Can you work these out from the model? Positions are in its coordinate system, mm. A direction names the side the tool comes from. Coordinates: 2 decimals unless noted, no trailing zeros. Loops run counter-clockwise (first coordinate to the right, second up) from the corner with the lowest first, then second, coordinate; pieces in that order, holes last. Notation, with made-up numbers: M -5.5,83 L 27.5,83 A22 ccw 27.5,112 Z; hole C 49,80.25 d11. An arc over 180 degrees is marked long. Answer as a JSON object with one key per item and string values. Group by question number.
Item 1: Suppose I cut it at A-A (y = 20). Write out the boundary of the cut face in (x, z).
Item 2: Which directions (+Z, -Z, +X, -X, +Y, -Y) give clear straight access to the entire face, cutting with the end or side of a thin tool? Please do faces 4 (the cylindrical face through (127.502, 170.354, -59.79)), 5 (the flat face through (220.5, 142, -60)), 6 (the cylindrical face through (414.343, 143.385, 10.77)).
Item 3: I'm going to push flat-ended pins straight in: pin 1 Ø11 at (x, y) = (260.5, 174.5) entering from +Z; pin 2 Ø6 at (x, y) = (451.5, 139) entering from +Z; pin 3 Ø2.5 at (x, y) = (231, 140.5) entering from -Z. Where does each tip first touch, or does it pass through?
Item 4: If I drill on line 1 (Y direction, x = 360, z = -56); line 2 (Y direction, x = 349.5, z = 58.75); line 3 (Y direction, x = 400, z = 7), over which ranges is the centre line in solid material (lowest first)?
Item 5: Suppose I cut it at B-B (z = 6). Count the separate pieces of the cut face and the enclosed holes in it, then the cut area to 3 significant figures.
Item 6: We'd pull the mould along X, two halves only. Please class faces 1 (the flat face through (0, 168, 1)), 2 (the flat face through (264, 172, -45)), 3 (the flat face through (138.5, 198, -60)): +X half, -X half, draft (parallel to the pull), parting line (faces both ways), or undercut.
```python
from build123d import *

# Parameters (mm, degrees)
SKETCH1_W                  = 555
SKETCH1_H                  = 340
BOSS_EXTRUDE1_DEPTH        = 75
SKETCH3_R                  = 35.3
CUT_EXTRUDE1_DEPTH         = 10
SKETCH5_R                  = 30
CUT_EXTRUDE2_DEPTH         = 110
SKETCH6_R                  = 27
CUT_EXTRUDE3_DEPTH         = 218
SKETCH7_W                  = 32
SKETCH7_H                  = 68
CUT_EXTRUDE4_DEPTH         = 30
SKETCH8_R                  = 5
CUT_EXTRUDE5_DEPTH         = 23
LPATTERN1_COUNT            = 2
LPATTERN1_PITCH            = 62
LPATTERN1_COUNT_DIR2       = 2
LPATTERN1_PITCH_DIR2       = 62
LPATTERN2_COUNT            = 6
LPATTERN2_PITCH            = 82
LPATTERN2_COPY_1_SKETCH_R  = 5
LPATTERN2_COPY_1_DEPTH     = 23
LPATTERN2_COPY_2_SKETCH_R  = 5
LPATTERN2_COPY_2_DEPTH     = 23
LPATTERN2_COPY_3_SKETCH_R  = 5
LPATTERN2_COPY_3_DEPTH     = 23
LPATTERN2_COPY_4_SKETCH_R  = 5
LPATTERN2_COPY_4_DEPTH     = 23
LPATTERN2_COPY_5_SKETCH_R  = 5
LPATTERN2_COPY_5_DEPTH     = 23
LPATTERN2_COPY_6_SKETCH_R  = 5
LPATTERN2_COPY_6_DEPTH     = 23
LPATTERN2_COPY_7_SKETCH_R  = 5
LPATTERN2_COPY_7_DEPTH     = 23
LPATTERN2_COPY_8_SKETCH_R  = 5
LPATTERN2_COPY_8_DEPTH     = 23
LPATTERN2_COPY_9_SKETCH_R  = 5
LPATTERN2_COPY_9_DEPTH     = 23
LPATTERN2_COPY_10_SKETCH_R = 5
LPATTERN2_COPY_10_DEPTH    = 23
LPATTERN2_COPY_11_SKETCH_R = 5
LPATTERN2_COPY_11_DEPTH    = 23
LPATTERN2_COPY_12_SKETCH_R = 5
LPATTERN2_COPY_12_DEPTH    = 23
LPATTERN2_COPY_13_SKETCH_R = 5
LPATTERN2_COPY_13_DEPTH    = 23
LPATTERN2_COPY_14_SKETCH_R = 5
LPATTERN2_COPY_14_DEPTH    = 23
LPATTERN2_COPY_15_SKETCH_R = 5
LPATTERN2_COPY_15_DEPTH    = 23
SKETCH9_R                  = 9.5
CUT_EXTRUDE6_DEPTH         = 151
LPATTERN3_COUNT            = 7
LPATTERN3_PITCH            = 82
LPATTERN3_COUNT_DIR2       = 2
LPATTERN3_PITCH_DIR2       = 150
SKETCH14_R                 = 8
CUT_EXTRUDE7_DEPTH         = 556
LPATTERN4_COUNT            = 4
LPATTERN4_PITCH            = 100
FILLET1_R                  = 3


with BuildPart() as part:
    # Sketch1 → Boss-Extrude1 (new body, symmetric)
    with BuildSketch(Plane.XY):
        with Locations((277.5, 170)):
            Rectangle(SKETCH1_W, SKETCH1_H)
    extrude(amount=BOSS_EXTRUDE1_DEPTH, both=True)

    # Sketch3 → Cut-Extrude1 (cut)
    with BuildSketch(Plane.XY.offset(75)):
        with Locations((72.5, 170)):
            Circle(SKETCH3_R)
    cut_extrude1 = extrude(amount=-CUT_EXTRUDE1_DEPTH, mode=Mode.SUBTRACT)

    # Sketch5 → Cut-Extrude2 (cut)
    with BuildSketch(Plane.XY.offset(65)):
        with Locations((72.5, 170)):
            Circle(SKETCH5_R)
    cut_extrude2 = extrude(amount=-CUT_EXTRUDE2_DEPTH, mode=Mode.SUBTRACT)

    # Sketch6 → Cut-Extrude3 (cut)
    with BuildSketch(Plane.XY.offset(-45)):
        with Locations((72.5, 170)):
            Circle(SKETCH6_R)
    cut_extrude3 = extrude(amount=-CUT_EXTRUDE3_DEPTH, mode=Mode.SUBTRACT)

    # Sketch7 → Cut-Extrude4 (cut)
    with BuildSketch(Plane(origin=(0, 0, -75), x_dir=(-1, 0, 0), z_dir=(0, 0, -1))):
        with Locations((-72.5, 170)):
            Rectangle(SKETCH7_W, SKETCH7_H)
    cut_extrude4 = extrude(amount=-CUT_EXTRUDE4_DEPTH, mode=Mode.SUBTRACT)

    # Sketch8 → Cut-Extrude5 (cut)
    with BuildSketch(Plane.XY.offset(75)):
        with Locations((41.5, 201)):
            Circle(SKETCH8_R)
    cut_extrude5 = extrude(amount=-CUT_EXTRUDE5_DEPTH, mode=Mode.SUBTRACT)

    # LPattern1: Cut-Extrude5 2 × 2
    with Locations(*[(i * LPATTERN1_PITCH, -j * LPATTERN1_PITCH_DIR2, 0) for i in range(LPATTERN1_COUNT) for j in range(LPATTERN1_COUNT_DIR2) if (i, j) != (0, 0)]):
        add(cut_extrude5, mode=Mode.SUBTRACT)

    # LPattern2: Cut-Extrude1, Cut-Extrude2, Cut-Extrude3, Cut-Extrude4, Cut-Extrude5 ×6
    with Locations(*[(i * LPATTERN2_PITCH, 0, 0) for i in range(1, LPATTERN2_COUNT)]):
        add(cut_extrude1, mode=Mode.SUBTRACT)
        add(cut_extrude2, mode=Mode.SUBTRACT)
        add(cut_extrude3, mode=Mode.SUBTRACT)
        add(cut_extrude4, mode=Mode.SUBTRACT)
        add(cut_extrude5, mode=Mode.SUBTRACT)

    # LPattern2 copy 1 sketch → LPattern2 copy 1 (cut)
    with BuildSketch(Plane(origin=(82, -62, 75), x_dir=(1, 0, 0), z_dir=(0, 0, 1))):
        with Locations((41.5, 201)):
            Circle(LPATTERN2_COPY_1_SKETCH_R)
    extrude(amount=-LPATTERN2_COPY_1_DEPTH, mode=Mode.SUBTRACT)

    # LPattern2 copy 2 sketch → LPattern2 copy 2 (cut)
    with BuildSketch(Plane(origin=(164, -62, 75), x_dir=(1, 0, 0), z_dir=(0, 0, 1))):
        with Locations((41.5, 201)):
            Circle(LPATTERN2_COPY_2_SKETCH_R)
    extrude(amount=-LPATTERN2_COPY_2_DEPTH, mode=Mode.SUBTRACT)

    # LPattern2 copy 3 sketch → LPattern2 copy 3 (cut)
    with BuildSketch(Plane(origin=(246, -62, 75), x_dir=(1, 0, 0), z_dir=(0, 0, 1))):
        with Locations((41.5, 201)):
            Circle(LPATTERN2_COPY_3_SKETCH_R)
    extrude(amount=-LPATTERN2_COPY_3_DEPTH, mode=Mode.SUBTRACT)

    # LPattern2 copy 4 sketch → LPattern2 copy 4 (cut)
    with BuildSketch(Plane(origin=(328, -62, 75), x_dir=(1, 0, 0), z_dir=(0, 0, 1))):
        with Locations((41.5, 201)):
            Circle(LPATTERN2_COPY_4_SKETCH_R)
    extrude(amount=-LPATTERN2_COPY_4_DEPTH, mode=Mode.SUBTRACT)

    # LPattern2 copy 5 sketch → LPattern2 copy 5 (cut)
    with BuildSketch(Plane(origin=(410, -62, 75), x_dir=(1, 0, 0), z_dir=(0, 0, 1))):
        with Locations((41.5, 201)):
            Circle(LPATTERN2_COPY_5_SKETCH_R)
    extrude(amount=-LPATTERN2_COPY_5_DEPTH, mode=Mode.SUBTRACT)

    # LPattern2 copy 6 sketch → LPattern2 copy 6 (cut)
    with BuildSketch(Plane(origin=(144, 0, 75), x_dir=(1, 0, 0), z_dir=(0, 0, 1))):
        with Locations((41.5, 201)):
            Circle(LPATTERN2_COPY_6_SKETCH_R)
    extrude(amount=-LPATTERN2_COPY_6_DEPTH, mode=Mode.SUBTRACT)

    # LPattern2 copy 7 sketch → LPattern2 copy 7 (cut)
    with BuildSketch(Plane(origin=(226, 0, 75), x_dir=(1, 0, 0), z_dir=(0, 0, 1))):
        with Locations((41.5, 201)):
            Circle(LPATTERN2_COPY_7_SKETCH_R)
    extrude(amount=-LPATTERN2_COPY_7_DEPTH, mode=Mode.SUBTRACT)

    # LPattern2 copy 8 sketch → LPattern2 copy 8 (cut)
    with BuildSketch(Plane(origin=(308, 0, 75), x_dir=(1, 0, 0), z_dir=(0, 0, 1))):
        with Locations((41.5, 201)):
            Circle(LPATTERN2_COPY_8_SKETCH_R)
    extrude(amount=-LPATTERN2_COPY_8_DEPTH, mode=Mode.SUBTRACT)

    # LPattern2 copy 9 sketch → LPattern2 copy 9 (cut)
    with BuildSketch(Plane(origin=(390, 0, 75), x_dir=(1, 0, 0), z_dir=(0, 0, 1))):
        with Locations((41.5, 201)):
            Circle(LPATTERN2_COPY_9_SKETCH_R)
    extrude(amount=-LPATTERN2_COPY_9_DEPTH, mode=Mode.SUBTRACT)

    # LPattern2 copy 10 sketch → LPattern2 copy 10 (cut)
    with BuildSketch(Plane(origin=(472, 0, 75), x_dir=(1, 0, 0), z_dir=(0, 0, 1))):
        with Locations((41.5, 201)):
            Circle(LPATTERN2_COPY_10_SKETCH_R)
    extrude(amount=-LPATTERN2_COPY_10_DEPTH, mode=Mode.SUBTRACT)

    # LPattern2 copy 11 sketch → LPattern2 copy 11 (cut)
    with BuildSketch(Plane(origin=(144, -62, 75), x_dir=(1, 0, 0), z_dir=(0, 0, 1))):
        with Locations((41.5, 201)):
            Circle(LPATTERN2_COPY_11_SKETCH_R)
    extrude(amount=-LPATTERN2_COPY_11_DEPTH, mode=Mode.SUBTRACT)

    # LPattern2 copy 12 sketch → LPattern2 copy 12 (cut)
    with BuildSketch(Plane(origin=(226, -62, 75), x_dir=(1, 0, 0), z_dir=(0, 0, 1))):
        with Locations((41.5, 201)):
            Circle(LPATTERN2_COPY_12_SKETCH_R)
    extrude(amount=-LPATTERN2_COPY_12_DEPTH, mode=Mode.SUBTRACT)

    # LPattern2 copy 13 sketch → LPattern2 copy 13 (cut)
    with BuildSketch(Plane(origin=(308, -62, 75), x_dir=(1, 0, 0), z_dir=(0, 0, 1))):
        with Locations((41.5, 201)):
            Circle(LPATTERN2_COPY_13_SKETCH_R)
    extrude(amount=-LPATTERN2_COPY_13_DEPTH, mode=Mode.SUBTRACT)

    # LPattern2 copy 14 sketch → LPattern2 copy 14 (cut)
    with BuildSketch(Plane(origin=(390, -62, 75), x_dir=(1, 0, 0), z_dir=(0, 0, 1))):
        with Locations((41.5, 201)):
            Circle(LPATTERN2_COPY_14_SKETCH_R)
    extrude(amount=-LPATTERN2_COPY_14_DEPTH, mode=Mode.SUBTRACT)

    # LPattern2 copy 15 sketch → LPattern2 copy 15 (cut)
    with BuildSketch(Plane(origin=(472, -62, 75), x_dir=(1, 0, 0), z_dir=(0, 0, 1))):
        with Locations((41.5, 201)):
            Circle(LPATTERN2_COPY_15_SKETCH_R)
    extrude(amount=-LPATTERN2_COPY_15_DEPTH, mode=Mode.SUBTRACT)

    # Sketch9 → Cut-Extrude6 (cut, through all)
    with BuildSketch(Plane.XY.offset(75)):
        with Locations((31.5, 245)):
            Circle(SKETCH9_R)
    cut_extrude6 = extrude(amount=-CUT_EXTRUDE6_DEPTH, mode=Mode.SUBTRACT)

    # LPattern3: Cut-Extrude6 7 × 2
    with Locations(*[(i * LPATTERN3_PITCH, -j * LPATTERN3_PITCH_DIR2, 0) for i in range(LPATTERN3_COUNT) for j in range(LPATTERN3_COUNT_DIR2) if (i, j) != (0, 0)]):
        add(cut_extrude6, mode=Mode.SUBTRACT)

    # Sketch14 → Cut-Extrude7 (cut, through all)
    with BuildSketch(Plane(origin=(555, 0, 0), x_dir=(0, 0, -1), z_dir=(1, 0, 0))):
        with Locations((-50, 20)):
            Circle(SKETCH14_R)
    cut_extrude7 = extrude(amount=-CUT_EXTRUDE7_DEPTH, mode=Mode.SUBTRACT)

    # LPattern4: Cut-Extrude7 ×4
    with Locations(*[(0, i * LPATTERN4_PITCH, 0) for i in range(1, LPATTERN4_COUNT)]):
        add(cut_extrude7, mode=Mode.SUBTRACT)

    # Fillet1
    fillet1_edges = [part.edges().sort_by_distance(p)[0] for p in [
        (555, 170, 75),
        (277.5, 340, 75),
        (0, 170, 75),
        (277.5, 340, -75),
        (555, 170, -75),
        (277.5, 0, -75),
        (0, 170, -75),
        (0, 340, 0),
        (555, 340, 0),
        (555, 0, 0),
        (0, 0, 0),
        (277.5, 0, 75),
    ]]
    fillet(fillet1_edges, radius=FILLET1_R)


solid = part.part
```
From the geometry:
{
 "1": {"outline": "M 0,-72 A3 ccw 3,-75 L 552,-75 A3 ccw 555,-72 L 555,42 L 0,42 Z; M 0,58 L 555,58 L 555,72 A3 ccw 552,75 L 3,75 A3 ccw 0,72 Z"},
 "2": {"face 4": "+Z, -Z", "face 5": "-Z", "face 6": "+Z"},
 "3": {"pin 1": "z = -45", "pin 2": "z = 52", "pin 3": "z = -45"},
 "4": {"line 1": "0 to 85.51, 104.49 to 235.51, 254.49 to 340", "line 2": "0 to 134, 144 to 196, 206 to 340", "line 3": "0 to 140, 200 to 340"},
 "5": {"separate pieces": "1", "enclosed holes": "20", "area": "168,000 mm2"},
 "6": {"face 1": "-X half", "face 2": "undercut", "face 3": "undercut"}
}
